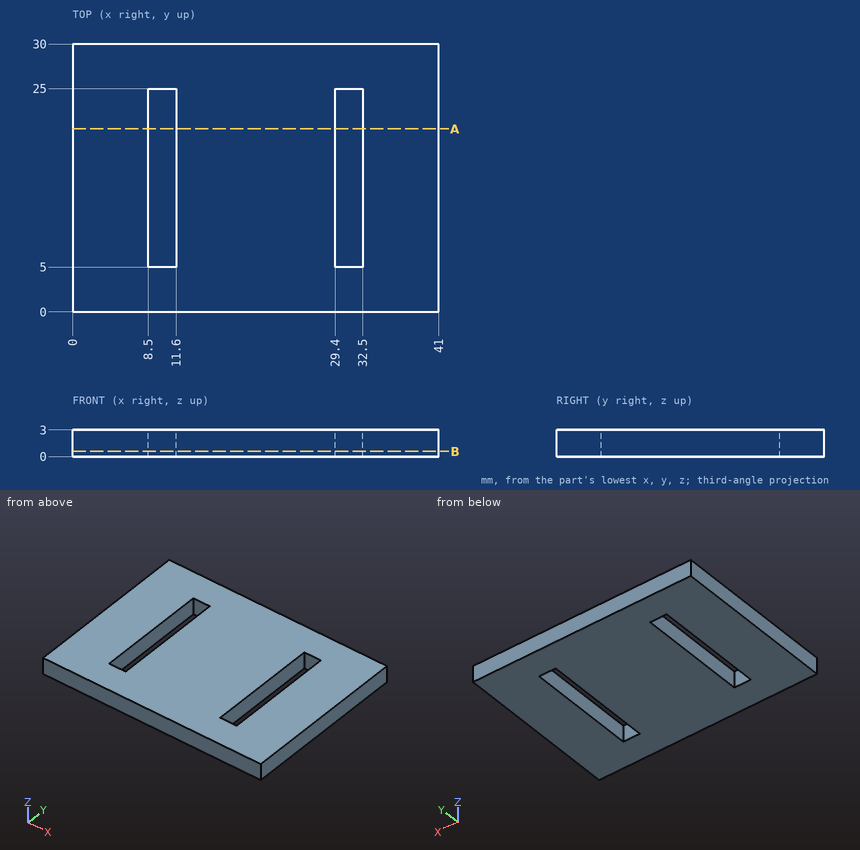
Check sheet for the drawn part. Datum: minimum x, y, z corner. Units: mm. Round coordinates to 2 decimals unless told otherwise and drop trailing zeros. Order: outer loops, then holes, each group sorted by start corner. A loop starts at its lowest first (then second) coordinate and runs counter-clockwise, first axis right, second up.
(1) Scan lines: probe 1 along X at (y, z) = (18.25, 2.5); probe 2 along Y at (x, z) = (31.5, 0.7). Record each from-to range of solid material in increasing order.
(2) Go/stop test with a flat-tipped pin: P1, Ø0.9, axis at y = 10.5, z = 2, coming from the -X side. Record where the tip stops, or that it passes through.
(3) Cross-section at B-B, the plane z = 0.6. Enter the section's corners in (x, y), and give its area (3 significant figures).
(4) Cross-section at A-A, the plane y = 20.5. Enter the section's corners in (x, z).
Check sheet entries:
1. probe 1: x = 0 to 8.5, 11.6 to 29.4, 32.5 to 41
1. probe 2: y = 0 to 5, 25 to 30
2. P1: stops at x = 0
3. outline: (0, 0) - (41, 0) - (41, 30) - (0, 30) - close; hole (8.5, 5) - (11.6, 5) - (11.6, 25) - (8.5, 25) - close; hole (29.4, 5) - (32.5, 5) - (32.5, 25) - (29.4, 25) - close
3. area: 1,110 mm2
4. outline: (0, 0) - (8.5, 0) - (8.5, 3) - (0, 3) - close; (11.6, 0) - (29.4, 0) - (29.4, 3) - (11.6, 3) - close; (32.5, 0) - (41, 0) - (41, 3) - (32.5, 3) - close
